from build123d import *

# Parameters (mm, degrees)
F0_R     = 3.683
F1_DEPTH = 19.812
F2_W     = 2.794
F2_H     = 2.1717
F3_DEPTH = 25.4
F4_R     = 0.381
F5_R     = 7.2136
F6_DEPTH = 12.7
F7_R     = 2.54
F8_R     = 0.635


with BuildPart() as f1:
    # F0 (on Top) → F1 (new body)
    with BuildSketch(Plane.XY):
        Circle(F0_R)
    extrude(amount=F1_DEPTH)

    # F2 (on face) → F3 (cut)
    with BuildSketch(Plane.XY.offset(19.812)):
        with Locations((0, -2.59715)):
            Rectangle(F2_W, F2_H)
    extrude(amount=-F3_DEPTH, mode=Mode.SUBTRACT)

    # F4
    f4_edges = [f1.edges().sort_by_distance(p)[0] for p in [
        (1.397, -3.407768, 9.906),
        (-1.397, -3.407768, 9.906),
    ]]
    fillet(f4_edges, radius=F4_R)

    # F5 (on face) → F6 (join)
    with BuildSketch(Plane(origin=(0, 0, 0), x_dir=(1, 0, 0), z_dir=(0, 0, -1))):
        Circle(F5_R)
    extrude(amount=F6_DEPTH)

    # F7
    f7_edges = [f1.edges().sort_by_distance(p)[0] for p in [
        (-7.2136, 0, -12.7),
    ]]
    fillet(f7_edges, radius=F7_R)

    # F8
    f8_edges = [f1.edges().sort_by_distance(p)[0] for p in [
        (-7.2136, 0, 0),
    ]]
    fillet(f8_edges, radius=F8_R)


solid = f1.part
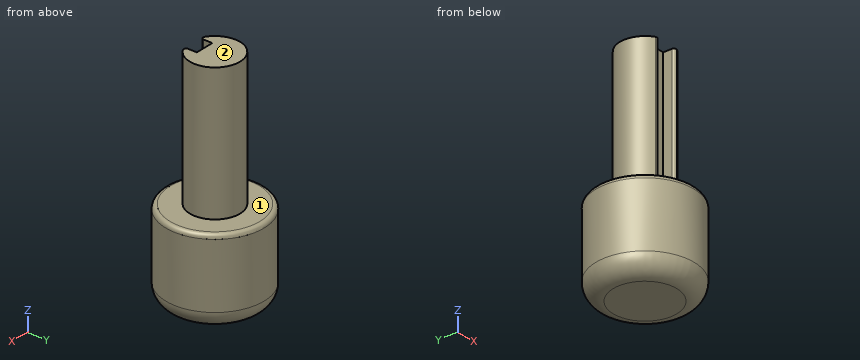
Could you check a few things on this model? Use its own coordinates, in mm. Face numbers are marked on the shaded views. A direction names the side the tool comes from. Round coordinates to 2 decimals unless told otherwise and drop trailing zeros. Write each loop counter-clockwise with the first axis right and the second up, starting at its lowest first coordinate (ties: lowest second). Pieces come first, ordered by that corner, then holes. Notation, with made-up numbers: (-10, 87) - (26, 87) arc R16 cw to (26, 110) - close; hole circle Ø6 at (81, 53.5). An arc over 180 degrees is marked (long way). Use a Markdown table: item, result.
Q1. I want a section at B-B (y = 0). List the corners of the cut face in (x, z) for me (3 decimals), plus the area to 3 significant figures.
Output values:
| item | result |
|---|---|
| outline | (-7.214, -10.16) arc R2.54 ccw to (-4.674, -12.7) - (4.674, -12.7) arc R2.54 ccw to (7.214, -10.16) - (7.214, -0.635) arc R0.635 ccw to (6.579, 0) - (3.683, 0) - (3.683, 19.812) - (-3.683, 19.812) - (-3.683, 0) - (-6.579, 0) arc R0.635 ccw to (-7.214, -0.635) - close |
| area | 326 mm2 |
Q2. I want a section at C-C (z = 2.5). List the corners of the cut face in (x, y) for me, plus the area to 3 significant figures.
Output values:
| item | result |
|---|---|
| outline | (-1.98, -3.1) arc R0.38 ccw to (-1.4, -2.78) - (-1.4, -1.51) - (1.4, -1.51) - (1.4, -2.78) arc R0.38 ccw to (1.98, -3.1) arc R3.68 ccw (long way) to start |
| area | 36.6 mm2 |
Q3. I want a section at D-D (z = -6). List the corners of the cut face in (x, y) for me.
Output values:
| item | result |
|---|---|
| outline | circle Ø14.43 at (0, 0) |
Q4. I want a section at A-A (x = 0). List the corners of the cut face in (y, z) for me (3 decimals), plus the area to 3 significant figures.
Output values:
| item | result |
|---|---|
| outline | (-7.214, -10.16) arc R2.54 ccw to (-4.674, -12.7) - (4.674, -12.7) arc R2.54 ccw to (7.214, -10.16) - (7.214, -0.635) arc R0.635 ccw to (6.579, 0) - (3.683, 0) - (3.683, 19.812) - (-1.511, 19.812) - (-1.511, 0) - (-6.579, 0) arc R0.635 ccw to (-7.214, -0.635) - close |
| area | 283 mm2 |
Q5. For pin 1 (1 mm diameter, centred on y = -2, z = 10.5, fed in from +X); pin 2 (1 mm diameter, centred on y = -2, z = 14.5, fed in from -X); pin 3 (2 mm diameter, centred on y = -1, z = 9.5, fed in from -X), each with a flat end and sliding along its axis, tell me the tip position at first contact or that it passes through.
Output values:
| item | result |
|---|---|
| pin 1 | x = 3.36 |
| pin 2 | x = -3.36 |
| pin 3 | x = -3.68 |
Q6. For the marked faces 1 and 2, which set-ups out of +Z, -Z, +X, -X, +Y, -Y let a thin tool reach every point of the face, with its end or its side?
Output values:
| item | result |
|---|---|
| face 1 | +Z |
| face 2 | +Z, +X, -X, +Y, -Y |
Q7. Please list where these lines run through material, in increasing order: L1, parallel to Z at x = 0.75, y = -2; L2, parallel to Y at x = 3, z = 16.5; L3, parallel to X at y = 1, z = 17.
Output values:
| item | result |
|---|---|
| L1 | -12.7 to 0 |
| L2 | -2.14 to 2.14 |
| L3 | -3.54 to 3.54 |
